Source: CAD feature listing. Evaluate the final solid. Frame: model axes, mm. Face numbers are marked on the shaded views. A direction names the side the tool comes from. Give positions to 0.01 mm unless a question says otherwise; leave off trailing zeros. Order: outer loops, then holes, each group sorted by start corner. A loop starts at its lowest first (then second) coordinate and runs counter-clockwise, first axis right, second up. Notation, with made-up numbers: M 1,86 L 13,86 A26 cw 13,111 Z; hole C 12,11 d7. An arc over 180 degrees is marked long. Return JSON: item names as keys, results as strings.
from build123d import *

# Parameters (mm, degrees)
F1_DEPTH = 19.05
F3_D     = 19.05
F5_DEPTH = 19.05


with BuildPart() as f1:
    # F0 (on Front) → F1 (new body)
    with BuildSketch(Plane.XZ):
        Polygon((176.9548937415, 719.3245387082), (-238.3473223164, 0), (-135.6944444544, 0), (270.4423360801, 703.4495387082), (242.9460295099, 719.3245387082), align=None)
    extrude(amount=F1_DEPTH)

    # F3 (through all)
    with Locations(Plane(origin=(0, 0, 0), x_dir=(1, 0, 0), z_dir=(0, 1, 0))):
        with Locations((17.6350068819, -354.4744000111)):
            Hole(F3_D / 2)

    # F4 (on Front) → F5 (join)
    with BuildSketch(Plane.XZ):
        Polygon((170.9644582182, 0), (273.6173360801, 0), (-141.6848799778, 719.3245387082), (-207.6760157462, 719.3245387082), (-235.1723223164, 703.4495387082), align=None)
    extrude(amount=-F5_DEPTH)


solid = f1.part
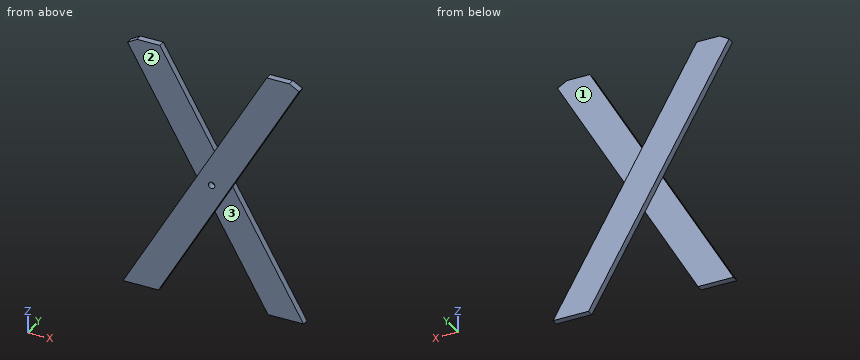
1. Section query C-C (z = 589). Return loops of the section in (x, y), then the cut area to 3 significant figures.
Evaluation:
{"outline": "M -169.09,0 L -66.44,0 L -66.44,19.05 L -169.09,19.05 Z; M 101.71,-19.05 L 204.36,-19.05 L 204.36,0 L 101.71,0 Z", "area": "3,910 mm^2"}
2. First-contact query: pin 1 (2 mm diameter, centred on y = 14, z = 486, fed in from +X); pin 2 (4 mm diameter, centred on x = -104, y = 4.5, fed in from +Z); pin 3 (9.5 mm diameter, centred on x = 14, z = 352, fed in from -Y). Flat tips, straight axial feed; report the tip coordinate or a pass-through.
Evaluation:
{"pin 1": "stops at x = -6.4", "pin 2": "stops at z = 657.52", "pin 3": "stops at y = 0"}
3. Section query B-B (y = -11). Return loops of the section in (x, z) (3 decimals).
Evaluation:
{"outline": "M -238.347,0 L -135.694,0 L 270.442,703.45 L 242.946,719.325 L 176.955,719.325 Z; hole C 17.635,354.474 d19.05"}
4. Section query A-A (x = 185). Return loops of the section in (y, z), then the cut area to 3 significant figures.
Evaluation:
{"outline": "M -19.05,555.46 L 0,555.46 L 0,719.32 L -19.05,719.32 Z; M 0,0 L 19.05,0 L 19.05,153.49 L 0,153.49 Z", "area": "6,050 mm^2"}
5. Ray query, probe 1 along Y at (x, z) = (90, 451.5); probe 2 along Y at (x, z) = (235, 45); probe 3 along X at (y, z) = (-15, 37.5). Return the intervals inside material, ascending.
Evaluation:
{"probe 1": "y = -19.05 to 0", "probe 2": "y = 0 to 19.05", "probe 3": "x = -216.7 to -114.04"}
6. Set-up query: the marked faces 1, 2 and 3. Return all of +Z, -Z, +X, -X, +Y, -Y with unobstructed straight access to the full face (end or side cutting, diameter ignored); none if empty.
Evaluation:
{"face 1": "+Z, +X, +Y", "face 2": "+Z, -X, -Y", "face 3": "-Z, +X, -Y"}
